```python
from build123d import *

# Parameters (mm, degrees)
F0_W     = 60
F0_H     = 60
F0_W_2   = 55
F0_H_2   = 55
F1_DEPTH = 500
F2_R     = 8.5
F3_DEPTH = 5
F4_R     = 8.5
F5_DEPTH = 5
F6_R     = 5.15
F7_DEPTH = 5
F8_R     = 5.15
F9_DEPTH = 5


with BuildPart() as f1:
    # F0 (on Top) → F1 (new body)
    with BuildSketch(Plane.XY):
        Rectangle(F0_W, F0_H)
        Rectangle(F0_W_2, F0_H_2, mode=Mode.SUBTRACT)
    extrude(amount=-F1_DEPTH)

    # F2 (on face) → F3 (cut)
    with BuildSketch(Plane.XZ.offset(30)):
        with Locations((0, -40)):
            Circle(F2_R)
        with Locations((0, -120)):
            Circle(F2_R)
    extrude(amount=-F3_DEPTH, mode=Mode.SUBTRACT)

    # F4 (on face) → F5 (cut)
    with BuildSketch(Plane.YZ.offset(30)):
        with Locations((0, -40)):
            Circle(F4_R)
        with Locations((0, -120)):
            Circle(F4_R)
    extrude(amount=-F5_DEPTH, mode=Mode.SUBTRACT)

    # F6 (on face) → F7 (cut)
    with BuildSketch(Plane(origin=(-30, 0, 0), x_dir=(0, -1, 0), z_dir=(-1, 0, 0))):
        with Locations((0, -40)):
            Circle(F6_R)
        with Locations((0, -120)):
            Circle(F6_R)
    extrude(amount=-F7_DEPTH, mode=Mode.SUBTRACT)

    # F8 (on face) → F9 (cut)
    with BuildSketch(Plane(origin=(0, 30, 0), x_dir=(-1, 0, 0), z_dir=(0, 1, 0))):
        with Locations((0, -40)):
            Circle(F8_R)
        with Locations((0, -120)):
            Circle(F8_R)
    extrude(amount=-F9_DEPTH, mode=Mode.SUBTRACT)


solid = f1.part
```
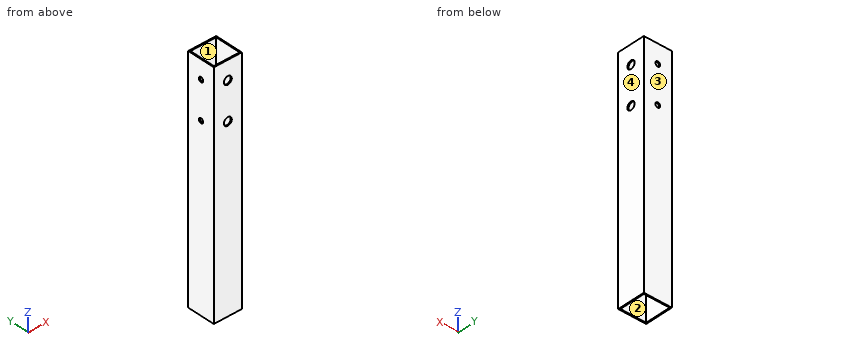
Check sheet for the modelled part. Datum: model origin and axes. Units: mm. Face numbers are marked on the shaded views. Give positions to 0.01 mm unless a question says otherwise; leave off trailing zeros. Order: outer loops, then holes, each group sorted by start corner. A loop starts at its lowest first (then second) coordinate and runs counter-clockwise, first axis right, second up. Notation, with made-up numbers: (16, 88) -> (51, 88) arc R30 cw to (51, 113) -> close; hole circle Ø5 at (62.5, 48.5). An arc over 180 degrees is marked (long way). Return JSON: item names as keys, results as strings.
1. Material ranges on probe 1 along Z at (x, y) = (0, -27.95); probe 2 along Y at (x, z) = (26.5, -248), recorded low to high. Write a range as [from, to].
From the geometry:
{"probe 1": "[-500, -128.5], [-111.5, -48.5], [-31.5, 0]", "probe 2": "[-30, -27.5], [27.5, 30]"}
2. Go/stop test with flat-tipped pins: P1, Ø13.5, axis at x = 0, z = -40, coming from the +Y side; P2, Ø13.5, axis at y = 0, z = -40, coming from the +X side; P3, Ø16.5, axis at x = 0, z = -120, coming from the -Y side. Record where each tip stops, or that it passes through.
From the geometry:
{"P1": "y = 30", "P2": "x = -27.5", "P3": "y = 27.5"}
3. Mould release check, pull along X, two halves, no side actions. Record for the marked faces 1, 2, 3 and 4: +X half, -X half, draft (parallel to the pull), parting line (faces both ways), or undercut.
From the geometry:
{"face 1": "undercut", "face 2": "undercut", "face 3": "draft", "face 4": "+X half"}
4. Cross-section at B-B, the plane x = 18.5. Record the cut outline in (y, z), plus the area to 3 significant figures.
From the geometry:
{"outline": "(-30, -500) -> (-27.5, -500) -> (-27.5, 0) -> (-30, 0) -> close; (27.5, -500) -> (30, -500) -> (30, 0) -> (27.5, 0) -> close", "area": "2,500 mm^2"}
5. Cross-section at D-D, the plane z = -329. Record the cut outline in (x, y), plus the area to 3 significant figures.
From the geometry:
{"outline": "(-30, -30) -> (30, -30) -> (30, 30) -> (-30, 30) -> close; hole (-27.5, -27.5) -> (27.5, -27.5) -> (27.5, 27.5) -> (-27.5, 27.5) -> close", "area": "575 mm^2"}
6. Cross-section at A-A, the plane z = -40. Record the cut outline in (x, y), plus the area to 4 significant figures.
From the geometry:
{"outline": "(-30, -30) -> (-8.5, -30) -> (-8.5, -27.5) -> (-27.5, -27.5) -> (-27.5, -5.15) -> (-30, -5.15) -> close; (-30, 5.15) -> (-27.5, 5.15) -> (-27.5, 27.5) -> (-5.15, 27.5) -> (-5.15, 30) -> (-30, 30) -> close; (5.15, 27.5) -> (27.5, 27.5) -> (27.5, 8.5) -> (30, 8.5) -> (30, 30) -> (5.15, 30) -> close; (8.5, -30) -> (30, -30) -> (30, -8.5) -> (27.5, -8.5) -> (27.5, -27.5) -> (8.5, -27.5) -> close", "area": "438.5 mm^2"}
